```python
from build123d import *

# Parameters (mm, degrees)
F1_DEPTH = 500
F2_R     = 1.5


with BuildPart() as f1:
    # F0 (on Front) → F1 (new body)
    with BuildSketch(Plane.XZ):
        Polygon((-7.46, 9.1), (-6.39934, 9.1), (-2.84, 9.1), (-3.74, 10), (-10, 10), (-10, 3.74), (-9.1, 2.84), (-9.1, 6.39934), (-9.1, 7.444134), (-9.124691, 7.46934), (-9.1, 9.1), align=None)
        Polygon((-7.399089, 8.459749), (-6.39934, 7.46), (-6.39934, 9.1), (-7.46, 9.1), (-7.110116, 8.742815), align=None)
        Polygon((-7.46, 6.39934), (-8.470702, 7.410042), (-8.774807, 7.112154), (-9.1, 7.444134), (-9.1, 6.39934), align=None)
        with BuildLine():
            ThreePointArc((-1.917323, 0.856663), (-1.729884, 1.190588), (-1.484924, 1.484924))
            Line((-1.484924, 1.484924), (-7.934896, 7.934896))
            Line((-7.934896, 7.934896), (-8.470702, 7.410042))
            Line((-8.470702, 7.410042), (-7.46, 6.39934))
            Line((-7.46, 6.39934), (-3.90066, 2.84))
            Line((-3.90066, 2.84), (-1.917323, 0.856663))
        make_face()
        with BuildLine():
            ThreePointArc((-1.484924, 1.484924), (-1.190588, 1.729884), (-0.856663, 1.917323))
            Line((-0.856663, 1.917323), (-2.84, 3.90066))
            Line((-2.84, 3.90066), (-6.39934, 7.46))
            Line((-6.39934, 7.46), (-7.399089, 8.459749))
            Line((-7.399089, 8.459749), (-7.934896, 7.934896))
            Line((-7.934896, 7.934896), (-1.484924, 1.484924))
        make_face()
        with BuildLine():
            ThreePointArc((0.856663, 1.917323), (1.484924, 1.484924), (1.917323, 0.856663))
            Line((1.917323, 0.856663), (3.90066, 2.84))
            Line((3.90066, 2.84), (7.46, 6.39934))
            Line((7.46, 6.39934), (9.1, 6.39934))
            Line((9.1, 6.39934), (9.1, 2.84))
            Line((9.1, 2.84), (10, 3.74))
            Line((10, 3.74), (10, 10))
            Line((10, 10), (3.74, 10))
            Line((3.74, 10), (2.84, 9.1))
            Line((2.84, 9.1), (6.39934, 9.1))
            Line((6.39934, 9.1), (6.39934, 7.46))
            Line((6.39934, 7.46), (2.84, 3.90066))
            Line((2.84, 3.90066), (0.856663, 1.917323))
        make_face()
        Polygon((7.112154, 8.774807), (7.46934, 9.124691), (9.1, 9.1), (9.1, 7.46), (8.742815, 7.110116), align=None, mode=Mode.SUBTRACT)
        with BuildLine():
            ThreePointArc((1.917323, 0.856663), (2.053823, 0.437962), (2.1, 0))
            ThreePointArc((2.1, 0), (2.053823, -0.437962), (1.917323, -0.856663))
            Line((1.917323, -0.856663), (3.90066, -2.84))
            Line((3.90066, -2.84), (3.90066, 2.84))
            Line((3.90066, 2.84), (1.917323, 0.856663))
        make_face()
        with BuildLine():
            ThreePointArc((-0.856663, 1.917323), (0, 2.1), (0.856663, 1.917323))
            Line((0.856663, 1.917323), (2.84, 3.90066))
            Line((2.84, 3.90066), (-2.84, 3.90066))
            Line((-2.84, 3.90066), (-0.856663, 1.917323))
        make_face()
        with BuildLine():
            ThreePointArc((-1.917323, -0.856663), (-2.1, 0), (-1.917323, 0.856663))
            Line((-1.917323, 0.856663), (-3.90066, 2.84))
            Line((-3.90066, 2.84), (-3.90066, -2.84))
            Line((-3.90066, -2.84), (-1.917323, -0.856663))
        make_face()
        with BuildLine():
            Line((2.84, -3.90066), (0.856663, -1.917323))
            ThreePointArc((0.856663, -1.917323), (0, -2.1), (-0.856663, -1.917323))
            Line((-0.856663, -1.917323), (-2.84, -3.90066))
            Line((-2.84, -3.90066), (2.84, -3.90066))
        make_face()
        with BuildLine():
            Line((-2.84, -3.90066), (-0.856663, -1.917323))
            ThreePointArc((-0.856663, -1.917323), (-1.190588, -1.729884), (-1.484924, -1.484924))
            Line((-1.484924, -1.484924), (-7.934896, -7.934896))
            Line((-7.934896, -7.934896), (-7.410042, -8.470702))
            Line((-7.410042, -8.470702), (-6.39934, -7.46))
            Line((-6.39934, -7.46), (-2.84, -3.90066))
        make_face()
        with BuildLine():
            Line((-7.934896, -7.934896), (-1.484924, -1.484924))
            ThreePointArc((-1.484924, -1.484924), (-1.729884, -1.190588), (-1.917323, -0.856663))
            Line((-1.917323, -0.856663), (-3.90066, -2.84))
            Line((-3.90066, -2.84), (-7.46, -6.39934))
            Line((-7.46, -6.39934), (-8.459749, -7.399089))
            Line((-8.459749, -7.399089), (-7.934896, -7.934896))
        make_face()
        with BuildLine():
            Line((7.934896, -7.934896), (1.484924, -1.484924))
            ThreePointArc((1.484924, -1.484924), (1.190588, -1.729884), (0.856663, -1.917323))
            Line((0.856663, -1.917323), (2.84, -3.90066))
            Line((2.84, -3.90066), (6.39934, -7.46))
            Line((6.39934, -7.46), (7.399089, -8.459749))
            Line((7.399089, -8.459749), (7.934896, -7.934896))
        make_face()
        with BuildLine():
            Line((3.90066, -2.84), (1.917323, -0.856663))
            ThreePointArc((1.917323, -0.856663), (1.729884, -1.190588), (1.484924, -1.484924))
            Line((1.484924, -1.484924), (7.934896, -7.934896))
            Line((7.934896, -7.934896), (8.470702, -7.410042))
            Line((8.470702, -7.410042), (7.46, -6.39934))
            Line((7.46, -6.39934), (3.90066, -2.84))
        make_face()
        Polygon((9.1, -2.84), (9.1, -6.39934), (9.1, -7.444134), (9.124691, -7.46934), (9.1, -9.1), (7.46, -9.1), (6.39934, -9.1), (2.84, -9.1), (3.74, -10), (10, -10), (10, -3.74), align=None)
        Polygon((9.1, -6.39934), (7.46, -6.39934), (8.470702, -7.410042), (8.774807, -7.112154), (9.1, -7.444134), align=None)
        Polygon((7.110116, -8.742815), (7.399089, -8.459749), (6.39934, -7.46), (6.39934, -9.1), (7.46, -9.1), align=None)
        Polygon((-2.84, -9.1), (-6.39934, -9.1), (-7.444134, -9.1), (-7.46934, -9.124691), (-9.1, -9.1), (-9.1, -7.46), (-9.1, -6.39934), (-9.1, -2.84), (-10, -3.74), (-10, -10), (-3.74, -10), align=None)
        Polygon((-6.39934, -9.1), (-6.39934, -7.46), (-7.410042, -8.470702), (-7.112154, -8.774807), (-7.444134, -9.1), align=None)
        Polygon((-8.742815, -7.110116), (-8.459749, -7.399089), (-7.46, -6.39934), (-9.1, -6.39934), (-9.1, -7.46), align=None)
    extrude(amount=F1_DEPTH)

    # F2
    f2_edges = [f1.edges().sort_by_distance(p)[0] for p in [
        (10, -250, 10),
        (-10, -250, 10),
        (-10, -250, -10),
        (10, -250, -10),
    ]]
    fillet(f2_edges, radius=F2_R)


solid = f1.part
```
Could you check a few things on this model? Use its own coordinates, in mm. Coordinates: 2 decimals unless noted, no trailing zeros. Use a Markdown table: item, result. Add a question column.
Q1. I want a section at A-A on y = -275. Give the number of separate pieces and of enclosed holes in the cut face, then the cut area to 3 significant figures.
Q2. I'm going to push flat-ended pins straight in: pin 1 (2 mm diameter, centred on y = -278, z = -0.5, fed in from +X); pin 2 (4.5 mm diameter, centred on y = -216.5, z = 0, fed in from -X). Where does each tip first touch, or does it pass through?
Q3. If I drill on L1, parallel to Z at x = 7.5, y = -358; L2, parallel to Z at x = 8, y = -157, over which ranges is the centre line in solid material (lowest first)?
Checked values:
| question | item | result |
|---|---|---|
| 1 | separate pieces | 1 |
| 1 | enclosed holes | 5 |
| 1 | area | 135 mm² |
| 2 | pin 1 | x = 3.9 |
| 2 | pin 2 | x = -3.9 |
| 3 | L1 | -10 to -9.1, -8.36 to -6.4, 6.4 to 8.38, 9.12 to 10 |
| 3 | L2 | -10 to -9.1, -7.87 to -6.4, 6.4 to 7.87, 9.12 to 10 |
